The figure shows three views and two pictorial views of one solid part (mm, origin at its lowest corner). Answer the questions. Coordinates: 2 decimals unless noted, no trailing zeros. Order: outer loops, then holes, each group sorted by start corner. A loop starts at its lowest first (then second) coordinate and runs counter-clockwise, first axis right, second up. Notation, with made-up numbers: (-25.5, 72.5) - (15.5, 72.5) arc R29 ccw to (15.5, 92.5) - close; hole circle Ø3 at (34, 77). An arc over 180 degrees is marked (long way). Use one line per item in the form item = value. Start each with the question number.
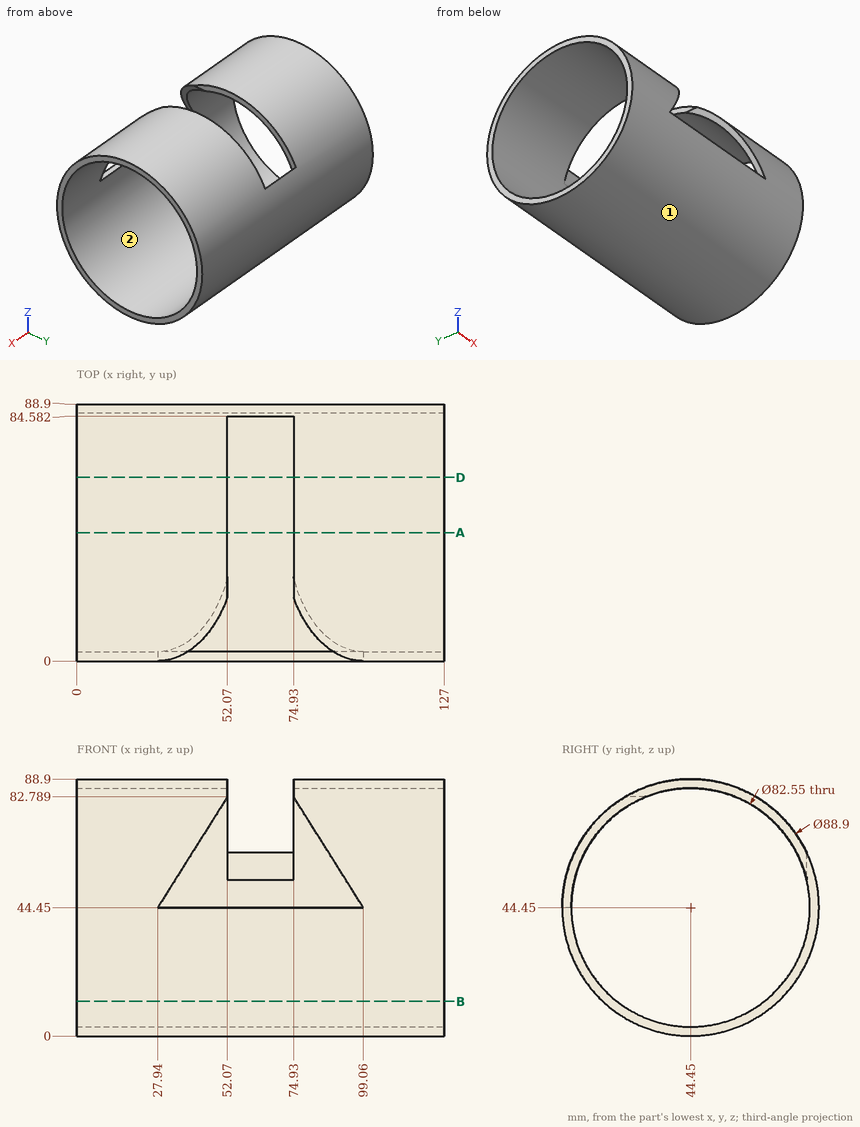
Q1. Given P1, Ø5, axis at x = 48, z = 72.5, coming from the +Y side; P2, Ø5, axis at x = 86, y = 22.5, coming from the +Z side; P3, Ø6, axis at x = 45.5, z = 75.5, coming from the +Y side; P4, Ø4, axis at x = 101, z = 42.5, coming from the +Y side, each flat-ended and moving along its own axis, determine where each tip first touches the part or whether it passes through.
Q2. Consider probe 1 along Y at (x, z) = (96, 44); probe 2 along Z at (x, y) = (27.5, 44.45) (1 decimal); probe 3 along X at (y, z) = (80, 67). Determine where each line is inside the solid, lowest interval first.
Q3. A cutting plane is placed at A-A (y = 44.45). Give the vertices of the cut face in (x, z) (1 decimal).
Q4. A cutting plane is placed at B-B (z = 12). Give the vertices of the cut face in (x, y), then the cut area to 3 significant figures.
Q5. For a pull along Y with two mould halves and no side action, classify the marked faces 1 and 2 as +Y half, -Y half, draft (parallel to the pull), parting line (faces both ways), or undercut.
Q6. A cutting plane is placed at D-D (y = 63.5). Give the vertices of the cut face in (x, z) (1 decimal).
Result sheet:
q1.P1 = 80.82
q1.P2 = 84.42
q1.P3 = 78.93
q1.P4 = 88.9
q2.probe_1 = 0 to 3.18, 85.72 to 88.9
q2.probe_2 = 0 to 3.2, 85.7 to 88.9
q2.probe_3 = 0 to 52.07, 74.93 to 127
q3.outline = (0, 0) - (127, 0) - (127, 3.2) - (0, 3.2) - close; (0, 85.7) - (52.1, 85.7) - (52.1, 88.9) - (0, 88.9) - close; (74.9, 85.7) - (127, 85.7) - (127, 88.9) - (74.9, 88.9) - close
q4.outline = (0, 14.07) - (127, 14.07) - (127, 18.94) - (0, 18.94) - close; (0, 69.96) - (127, 69.96) - (127, 74.83) - (0, 74.83) - close
q4.area = 1,240 mm^2
q5.face_1 = parting line
q5.face_2 = undercut
q6.outline = (0, 4.3) - (127, 4.3) - (127, 7.8) - (0, 7.8) - close; (0, 81.1) - (52.1, 81.1) - (52.1, 84.6) - (0, 84.6) - close; (74.9, 81.1) - (127, 81.1) - (127, 84.6) - (74.9, 84.6) - close
